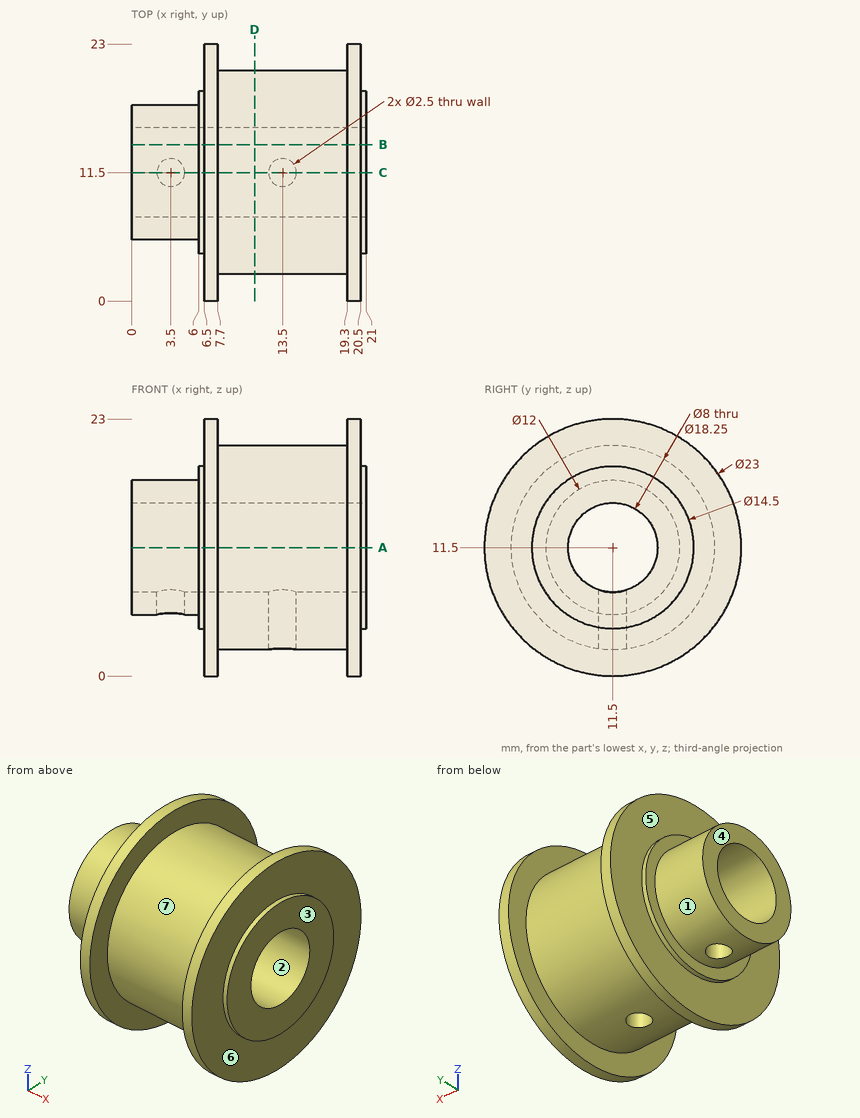
Here's the drawing with two shaded views (mm, measured from the low corner). I have some questions. A direction names the side the tool comes from. Coordinates: 2 decimals unless noted, no trailing zeros. Loops run counter-clockwise (first coordinate to the right, second up) from the corner with the lowest first, then second, coordinate; pieces in that order, holes last. Notation, with made-up numbers: M 43.25,36 L 100.25,36 A37 cw 100.25,73 Z; hole C 73,5.25 d3. An arc over 180 degrees is marked long. Put each result on its own line as item: value. Start each with the question number.
(1) Will these pins go through, and if not, where does the flat tip stop? pin 1 Ø3 at (x, y) = (13.5, 11.5) entering from -Z (3 decimals); pin 2 Ø1.5 at (x, z) = (12.5, 11) entering from -Y (3 decimals); pin 3 Ø5 at (y, z) = (11.5, 11.5) entering from -X; pin 4 Ø2 at (x, y) = (11.5, 19) entering from +Z.
(2) Imagine slicing it at A-A on z = 11.5. List the corners of the cut face in (x, y) for me (3 decimals).
(3) Imagine slicing it at B-B on y = 14. List the corners of the cut face in (x, z) for me, and give its area (3 significant figures).
(4) Imagine slicing it at C-C on y = 11.5. Give the number of separate pieces and of enclosed holes in the cut face, and give its area (3 significant figures).
(5) Which directions (+Z, -Z, +X, -X, +Y, -Y) give clear straight access to the entire face, cutting with the end or side of a thin tool? Please do the marked faces 4, 5, 6 and 7.
(6) I need wall thicknesses on probe 1 along X at (y, z) = (11.5, 6.2); probe 2 along Z at (x, y) = (11.5, 11.25); probe 3 along X at (y, z) = (11.5, 4.4). Which ranges of each line are inside material? Lowest first, please.
(7) Imagine slicing it at D-D on x = 11. List the corners of the cut face in (y, z) for me (3 decimals).
(8) We'd pull the mould along Y, two halves only. Please class the marked faces 1, 2 and 3: +Y half, -Y half, draft (parallel to the pull), parting line (faces both ways), or undercut.
Worked answers:
1. pin 1: stops at z = 2.375
1. pin 2: stops at y = 2.375
1. pin 3: passes through
1. pin 4: stops at z = 17.9
2. outline: M 0,5.5 L 6,5.5 L 6,4.25 L 6.5,4.25 L 6.5,0 L 7.7,0 L 7.7,2.375 L 19.3,2.375 L 19.3,0 L 20.5,0 L 20.5,4.25 L 21,4.25 L 21,7.5 L 0,7.5 Z; M 0,15.5 L 21,15.5 L 21,18.75 L 20.5,18.75 L 20.5,23 L 19.3,23 L 19.3,20.625 L 7.7,20.625 L 7.7,23 L 6.5,23 L 6.5,18.75 L 6,18.75 L 6,17.5 L 0,17.5 Z
3. outline: M 0,6.05 L 6,6.05 L 6,4.69 L 6.5,4.69 L 6.5,0.28 L 7.7,0.28 L 7.7,2.72 L 19.3,2.72 L 19.3,0.28 L 20.5,0.28 L 20.5,4.69 L 21,4.69 L 21,8.38 L 0,8.38 Z; M 0,14.62 L 21,14.62 L 21,18.31 L 20.5,18.31 L 20.5,22.72 L 19.3,22.72 L 19.3,20.28 L 7.7,20.28 L 7.7,22.72 L 6.5,22.72 L 6.5,18.31 L 6,18.31 L 6,16.95 L 0,16.95 Z
3. area: 205 mm2
4. separate pieces: 4
4. enclosed holes: 0
4. area: 168 mm2
5. face 4: +Z, -Z, -X, +Y, -Y
5. face 5: -X
5. face 6: +X
5. face 7: none
6. probe 1: x = 0 to 2.25, 4.75 to 12.25, 14.75 to 21
6. probe 2: z = 2.38 to 7.51, 15.49 to 20.62
6. probe 3: x = 6 to 12.25, 14.75 to 21
7. outline: C 11.5,11.5 d18.25; hole C 11.5,11.5 d8
8. face 1: parting line
8. face 2: undercut
8. face 3: draft
